The model under review builds one solid part; all positions refer to its coordinate system, in mm. Round coordinates to 2 decimals unless told otherwise and drop trailing zeros. Loops run counter-clockwise (first coordinate to the right, second up) from the corner with the lowest first, then second, coordinate; pieces in that order, holes last. Notation, with made-up numbers: M -28,-36 L 11,-36 A32 ccw 11,-8 Z; hole C 27.5,-10 d10. An arc over 180 degrees is marked long. Answer in a Markdown table with one row per item. Add a question column.
Autodesk Inventor part; units mm, degrees
ref_plane "Work Plane1" through (0, 3, -56.2) normal (0, 0, 1) x (1, 0, 0)
ref_plane "YZ Plane" through (0, 0, 0) normal (1, 0, 0) x (0, 1, 0)
ref_plane "XZ Plane" through (0, 0, 0) normal (0, 1, 0) x (-1, 0, 0)
sketch "Sketch1" plane through (0, 0, 0) normal (0, 1, 0) x (-1, 0, 0)
  line L0 (0, 0) -> (0, -112.4)
  line L1 (0, 0) -> (112.4, 0) construction
  line L2 (0, -112.4) -> (-61.993, -112.4)
  line L3 (0, -112.4) -> (61.993, -112.4) construction
  line L4 (0, 0) -> (-61.993, 0)
  line L5 (0, 0) -> (61.993, 0) construction
  line L6 (-61.993, -112.4) -> (-84.969, -89.424)
  line L7 (-61.993, -112.4) -> (-29.5, -112.4) construction
  line L8 (-61.993, 0) -> (-84.969, -22.976)
  line L9 (-61.993, 0) -> (-29.5, 0) construction
  line L10 (-84.969, -22.976) -> (-84.969, -89.424)
  line L11 (-84.969, -56.2) -> (-89.969, -56.2)
  line L12 (-84.969, -89.424) -> (-89.969, -56.2)
  line L13 (-84.969, -22.976) -> (-89.969, -56.2)
  line L14 (0, -112.4) -> (0, -109.6)
  line L15 (0, -109.6) -> (-5, -109.6)
  line L16 (-5, -109.6) -> (-5, -110.6)
  line L17 (-5, -110.6) -> (-15, -110.6)
  line L18 (-15, -110.6) -> (-15, -108.6)
  line L19 (-15, -108.6) -> (-5, -108.6)
  line L20 (-5, -108.6) -> (-5, -109.6)
  line L21 (-15, -75) -> (-15, -73)
  line L22 (-15, -73) -> (-5, -73)
  line L23 (-5, -75) -> (-15, -75)
  line L24 (-5, -74) -> (-5, -75)
  line L25 (-5, -73) -> (-5, -74)
  line L26 (-15, -39.4) -> (-15, -37.4)
  line L27 (-15, -37.4) -> (-5, -37.4)
  line L28 (-5, -39.4) -> (-15, -39.4)
  line L29 (-5, -38.4) -> (-5, -39.4)
  line L30 (-5, -37.4) -> (-5, -38.4)
  line L31 (-15, -3.8) -> (-15, -1.8)
  line L32 (-15, -1.8) -> (-5, -1.8)
  line L33 (-5, -3.8) -> (-15, -3.8)
  line L34 (-5, -2.8) -> (-5, -3.8)
  line L35 (-5, -1.8) -> (-5, -2.8)
  line L36 (-84.969, -89.424) -> (-77.898, -96.495)
  line L37 (-77.898, -96.495) -> (-74.3624, -92.9595)
  line L38 (-74.3624, -92.9595) -> (-75.0695, -92.2524)
  line L39 (-75.0695, -92.2524) -> (-67.9985, -85.1813)
  line L40 (-67.9985, -85.1813) -> (-66.5842, -86.5956)
  line L41 (-66.5842, -86.5956) -> (-73.6553, -93.6666)
  line L42 (-73.6553, -93.6666) -> (-74.3624, -92.9595)
  line L43 (-74.3624, -19.4405) -> (-75.0695, -20.1476)
  line L44 (-75.0695, -20.1476) -> (-67.9985, -27.2187)
  line L45 (-67.9985, -27.2187) -> (-66.5842, -25.8044)
  line L46 (-66.5842, -25.8044) -> (-73.6553, -18.7334)
  line L47 (-73.6553, -18.7334) -> (-74.3624, -19.4405)
  line L48 (-61.993, -112.4) -> (-54.8, -112.4)
  line L49 (-54.8, -112.4) -> (-54.8, -107.4)
  line L50 (-54.8, -107.4) -> (-55.8, -107.4)
  line L51 (-55.8, -107.4) -> (-55.8, -97.4)
  line L52 (-55.8, -97.4) -> (-53.8, -97.4)
  line L53 (-53.8, -97.4) -> (-53.8, -107.4)
  line L54 (-53.8, -107.4) -> (-54.8, -107.4)
  line L55 (-54.8, -5) -> (-55.8, -5)
  line L56 (-55.8, -5) -> (-55.8, -15)
  line L57 (-55.8, -15) -> (-53.8, -15)
  line L58 (-53.8, -15) -> (-53.8, -5)
  line L59 (-53.8, -5) -> (-54.8, -5)
  dimension "d0" = 112.4
  dimension "d1" = 90
  dimension "d2" = 61.993
  dimension "d3" = 180
  dimension "d4" = 61.993
  dimension "d5" = 180
  dimension "d24" = 32.493
  dimension "d25" = 225
  dimension "d26" = 32.493
  dimension "d27" = 225
  dimension "d28" = 5
  dimension "d29" = 2.8
  dimension "d30" = 5
  dimension "d31" = 1
  dimension "d32" = 10
  dimension "d33" = 2
  dimension "d34" = 10
  dimension "d35" = 90
  dimension "d38" = 35.6
  dimension "d43" = 10
  dimension "d44" = 5
  dimension "d45" = 1
  dimension "d46" = 10
  dimension "d47" = 2
  dimension "d57" = 7.193
  dimension "d58" = 5
  dimension "d59" = 90
  dimension "d60" = 1
  dimension "d61" = 10
  dimension "d62" = 2
  dimension "d63" = 10
  dimension "d64" = 90
extrude "Extrusion1" add sketch "Sketch1" along normal blind 3 contours L0 L2 L6 L10 L8 L4
ref_plane "Work Plane1" through (0, 3, -56.2) normal (0, 0, 1) x (1, 0, 0)
sketch "Sketch4" plane through (0, 3, -56.2) normal (0, 0, 1) x (1, 0, 0)
  line L0 (15, 0) -> (84.969, 0)
  line L1 (84.969, 0) -> (61.993, 0)
  line L2 (84.969, 0) -> (49.9845, 0)
  line L3 (61.993, 0) -> (0, 0)
  line L4 (49.9845, 0) -> (49.9845, 27.44)
  circle A0 centre (49.9845, 27.44) radius 34.3
  line L5 (49.9845, -6.86) -> (49.9845, 61.74)
  point P0 (0, -3)
  dimension "d53" = 34.9845
  dimension "d54" = 27.44
  dimension "d55" = 68.6
revolve "Revolution2" cut sketch "Sketch4" angle 360 about axis through (49.9845, 3, -56.2) along (0, 1, 0) picked at (38.3687, -1.2506) picked at (43.1245, 9.1467) contours L5 A0 L0 | L0 A0 L5 L4
sketch "Sketch6" plane through (0, 3, -56.2) normal (0, 0, 1) x (1, 0, 0)
  line L0 (15, 0) -> (84.969, 0)
  line L1 (84.969, 0) -> (61.993, 0)
  line L2 (84.969, 0) -> (49.9845, 0)
  line L3 (61.993, 0) -> (0, 0)
  line L4 (49.9845, 0) -> (49.9845, 27.44)
  circle A0 centre (49.9845, 27.44) radius 34.3
  line L5 (49.9845, -6.86) -> (49.9845, 61.74)
  circle A1 centre (49.9845, 27.44) radius 37.3
  line L6 (49.9845, -9.86) -> (49.9845, -3)
  line L7 (84.969, -3) -> (61.993, -3)
  line L8 (71.5413, -3) -> (28.4277, -3)
  point P0 (0, -3)
  point P1 (0, -3)
  point P2 (65.7926, -3)
  dimension "d70" = 34.9845
  dimension "d71" = 27.44
  dimension "d72" = 68.6
  dimension "d73" = 3
revolve "Revolution4" add sketch "Sketch6" angle 360 about axis through (49.9845, -3.86, -56.2) along (0, 1, 0) contours A0 L7 A1 L6
properties part number "PalmInsert"
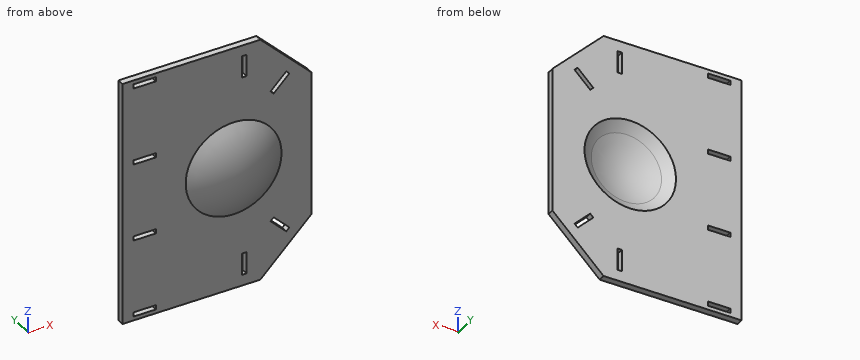
1. Take a section at C-C, the plane z = -46. State the section outline as (x, y) points.
2. Take a section at D-D, the plane y = 1.25. State how many separate pieces and enclosed holes the cut face has, and give its area (3 significant figures).
3. Take a section at A-A, the plane z = -9.5. State the section outline as (x, y) points, and give its area (3 significant figures).
4. To check wall thickness, follow probe 1 along Y at (x, z) = (51.5, -80); probe 2 along Z at (x, y) = (71, 1.75); probe 3 along Z at (x, y) = (46, 1.75). State the ranges of each line that lie inside material, in increasing order.
5. Take a section at B-B, the plane x = 45. State the section outline as (y, z) points.
6. For pin 1 Ø12 at (x, z) = (46.5, -45) entering from -Y; pin 2 Ø0.6 at (y, z) = (2, -2.5) entering from +X; pin 3 Ø2 at (x, z) = (40.5, -33) entering from -Y, all flat-tipped, find the tip position at first contact; note any pin that passes through.
Check sheet entries:
| question | item | result |
|---|---|---|
| 1 | outline | M 0,0 L 30.99,0 A35.88 ccw 68.98,0 L 84.97,0 L 84.97,3 L 67.86,3 A32.75 cw 32.11,3 L 0,3 Z |
| 2 | separate pieces | 1 |
| 2 | enclosed holes | 9 |
| 2 | area | 7,840 mm^2 |
| 3 | outline | M 0,0 L 53.8,0 L 53.8,3 L 0,3 Z; M 55.8,0 L 71.49,0 L 71.49,3 L 55.8,3 Z |
| 3 | area | 208 mm^2 |
| 4 | probe 1 | y = 0 to 3 |
| 4 | probe 2 | z = -103.39 to -91.01, -88.18 to -24.22, -21.39 to -9.01 |
| 4 | probe 3 | z = -112.4 to -74.57, -37.83 to 0 |
| 5 | outline | M 0,-112.4 L 3,-112.4 L 3,-76.17 A33.94 cw 3,-36.23 L 3,0 L 0,0 L 0,-35.23 A36.97 ccw 0,-77.17 Z |
| 6 | pin 1 | stops at y = -6.42 |
| 6 | pin 2 | stops at x = 64.79 |
| 6 | pin 3 | stops at y = 0 |
